Part model, mm, in its own coordinate system. Face numbers are marked on the shaded views. A direction names the side the tool comes from. Round coordinates to 2 decimals unless told otherwise and drop trailing zeros. Loops run counter-clockwise (first coordinate to the right, second up) from the corner with the lowest first, then second, coordinate; pieces in that order, holes last.
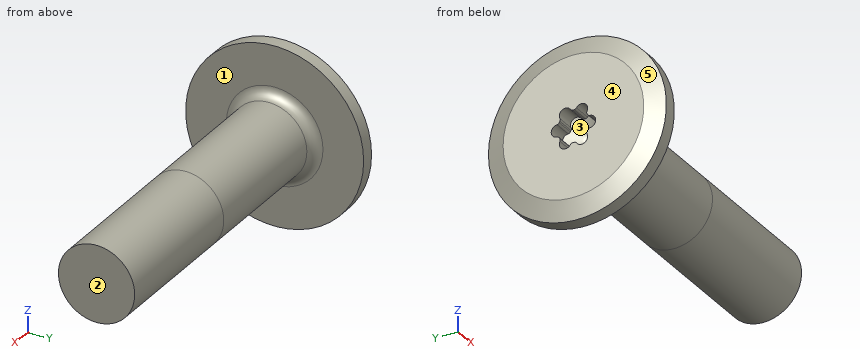
Autodesk Inventor part; units mm, degrees
ref_plane "YZ Plane" through (0, 0, 0) normal (1, 0, 0) x (0, 1, 0)
ref_plane "XZ Plane" through (0, 0, 0) normal (0, 1, 0) x (-1, 0, 0)
ref_plane "XY Plane" through (0, 0, 0) normal (0, 0, 1) x (1, 0, 0)
sketch "Sketch_1" plane through (0, 0, 0) normal (0, 0, 1) x (1, 0, 0)
  line L0 (6, 0) -> (0, 0)
  line L1 (-0.8, 0) -> (-0.8, 2.7673)
  line L2 (-0.8, 2.7673) -> (-0.5333, 3.5)
  line L3 (-0.5333, 3.5) -> (0, 3.5)
  line L4 (0, 3.5) -> (0, 1.9)
  arc A0 (0, 1.9) -> (0.4, 1.5) centre (0.4, 1.9) ccw
  line L5 (0.4, 1.5) -> (6, 1.5)
  line L6 (6, 1.5) -> (6, 0)
  line L7 (6, 0) -> (-0.8, 0)
  line L8 (0, 0) -> (-0.8, 0)
  dimension "d6" = 6
revolve "Revolution1" add sketch "Sketch_1" angle 360 about axis through (6, 0, 0) along (1, 0, 0)
sketch "Sketch_5" plane through (-0.05, 0, 0) normal (1, 0, 0) x (0, 0, -1)
  arc A0 (-0.6801, -0.1159) -> (-0.4404, -0.531) centre (-0.5499, -0.3175) ccw
  arc A1 (-0.341, -0.5357) -> (-0.4404, -0.531) centre (-0.3947, -0.62) ccw
  arc A2 (-0.341, -0.5357) -> (-0.2934, -0.5632) centre (0, 0) ccw
  arc A3 (-0.2397, -0.6469) -> (-0.2934, -0.5632) centre (-0.3396, -0.6519) ccw
  arc A4 (-0.2397, -0.6469) -> (0.2397, -0.6469) centre (0, -0.635) ccw
  arc A5 (0.2934, -0.5632) -> (0.2397, -0.6469) centre (0.3396, -0.6519) ccw
  arc A6 (0.2934, -0.5632) -> (0.341, -0.5357) centre (0, 0) ccw
  arc A7 (0.4404, -0.531) -> (0.341, -0.5357) centre (0.3947, -0.62) ccw
  arc A8 (0.4404, -0.531) -> (0.6801, -0.1159) centre (0.5499, -0.3175) ccw
  arc A9 (0.6344, -0.0275) -> (0.6801, -0.1159) centre (0.7343, -0.0318) ccw
  arc A10 (0.6344, -0.0275) -> (0.6344, 0.0275) centre (0, 0) ccw
  arc A11 (0.6801, 0.1159) -> (0.6344, 0.0275) centre (0.7343, 0.0318) ccw
  arc A12 (0.6801, 0.1159) -> (0.4404, 0.531) centre (0.5499, 0.3175) ccw
  arc A13 (0.341, 0.5357) -> (0.4404, 0.531) centre (0.3947, 0.62) ccw
  arc A14 (0.341, 0.5357) -> (0.2934, 0.5632) centre (0, 0) ccw
  arc A15 (0.2397, 0.6469) -> (0.2934, 0.5632) centre (0.3396, 0.6519) ccw
  arc A16 (0.2397, 0.6469) -> (-0.2397, 0.6469) centre (0, 0.635) ccw
  arc A17 (-0.2934, 0.5632) -> (-0.2397, 0.6469) centre (-0.3396, 0.6519) ccw
  arc A18 (-0.2934, 0.5632) -> (-0.341, 0.5357) centre (0, 0) ccw
  arc A19 (-0.4404, 0.531) -> (-0.341, 0.5357) centre (-0.3947, 0.62) ccw
  arc A20 (-0.4404, 0.531) -> (-0.6801, 0.1159) centre (-0.5499, 0.3175) ccw
  arc A21 (-0.6344, 0.0275) -> (-0.6801, 0.1159) centre (-0.7343, 0.0318) ccw
  arc A22 (-0.6344, 0.0275) -> (-0.6344, -0.0275) centre (0, 0) ccw
  arc A23 (-0.6801, -0.1159) -> (-0.6344, -0.0275) centre (-0.7343, -0.0318) ccw
extrude "Extrusion1" cut sketch "Sketch_5" against normal blind 0.75
sketch "Sketch_2" plane through (0, 0, 0) normal (0, 0, 1) x (1, 0, 0)
  line L0 (0.4552, 0) -> (0, 0)
  line L1 (-0.05, 0) -> (-0.05, 0.875)
  line L2 (-0.05, 0.875) -> (0.4552, 0)
  line L3 (0.4552, 0) -> (-0.05, 0)
revolve "Revolution2" cut sketch "Sketch_2" angle 360 about axis through (0.4552, 0, 0) along (1, 0, 0)
sketch "スケッチ4" plane through (6, 0, 0) normal (1, 0, 0) x (0, 0, -1)
  circle A0 centre (0, 0) radius 1.5
extrude "押し出し2" add sketch "スケッチ4" along normal blind 6
thread "Thread1"
properties part number "超極低頭ネジL12" material "ステンレス鋼"
1) Wall check: line 1 along X through (y, z) = (-2, 1); line 2 along Z through (x, y) = (4, 0); line 3 along Y through (x, z) = (4.25, 1.25). Give the ranges that are in metal, low to high.
Values:
line 1: x = -0.8 to 0
line 2: z = -1.5 to 1.5
line 3: y = -0.83 to 0.83
2) Tool access for the marked faces 1 and 2: list every direction of +Z, -Z, +X, -X, +Y, -Y with a clear straight run to the whole face (end or side of a thin tool).
Values:
face 1: +X
face 2: +Z, -Z, +X, +Y, -Y
3) Drop flat-ended pins along their axis: pin 1 Ø1.5 at (x, y) = (7.5, -0.5) entering from +Z; pin 2 Ø4 at (x, y) = (1, -3) entering from +Z; pin 3 Ø1.5 at (x, y) = (5, -0.5) entering from -Z. Give the stop position or say it passes through.
Values:
pin 1: stops at z = 1.5
pin 2: stops at z = 3.26
pin 3: stops at z = -1.5
4) Mould opens along Z. For the marked faces 3, 4 and 5 say: released by +Z, released by -Z, zero draft, split by the parting line, or undercut.
Values:
face 3: undercut
face 4: zero draft
face 5: split by the parting line
5) Slice it at A-A, the plane x = 8.25. Give the cut face in (y, z), then the cut area to 3 significant figures.
Values:
outline: circle Ø3 at (0, 0)
area: 7.07 mm2
